from build123d import *

# Parameters (mm, degrees)
F1_W = 69.838352
F1_H = 67.95083
F5_T = -2.54


with BuildPart() as f4:
    # F1 (on offset) → F4 section 0
    with BuildSketch(Plane.XY.offset(127)):
        Rectangle(F1_W, F1_H)
    # F3 (on offset) → F4 section 1
    with BuildSketch(Plane.XY.offset(-64.262)):
        Polygon((0, 23.29665), (-24.888797, 0), (0, -24.346344), (23.815714, 0), align=None)
    loft()

    # F5
    f5_openings = [f4.faces().sort_by_distance(p)[0] for p in [
        (0, 0, 127),
    ]]
    offset(amount=F5_T, openings=f5_openings)


solid = f4.part
Could you check a few things on this model? Use its own coordinates, in mm. Coordinates: 2 decimals unless noted, no trailing zeros.
1. I need wall thicknesses on L1, parallel to X at y = -16, z = -15.5; L2, parallel to Y at x = -25, z = 101; L3, parallel to X at y = -5.5, z = 18. Which ranges of each line are inside material? Lowest first, please.
2. For P1, Ø1, axis at x = 13, z = -6.5, coming from the -Y side; P2, Ø6, axis at x = -2.5, z = -15, coming from the +Y side; P3, Ø10, axis at y = -8, z = 15.5, coming from the -X side, each with a flat end and sliding along its axis, tell me the tip position at first contact or that it passes through.
3. We'd pull the mould along X, two halves only. Please class faces 1 (the face through (-1, 0, -61.722)), 2 (the face through (-33, 3, 127)): released by +X, released by -X, zero draft, split by the parting line, or undercut.
Computed values:
1. L1: x = -12.74 to -7.04, 11.44 to 14.31
1. L2: y = -29.8 to -27.22, 29.72 to 32.27
1. L3: x = -26.16 to -23.48, 19.58 to 22.26
2. P1: stops at y = -22.86
2. P2: stops at y = 24.35
2. P3: stops at x = -28.67
3. face 1: undercut
3. face 2: zero draft
